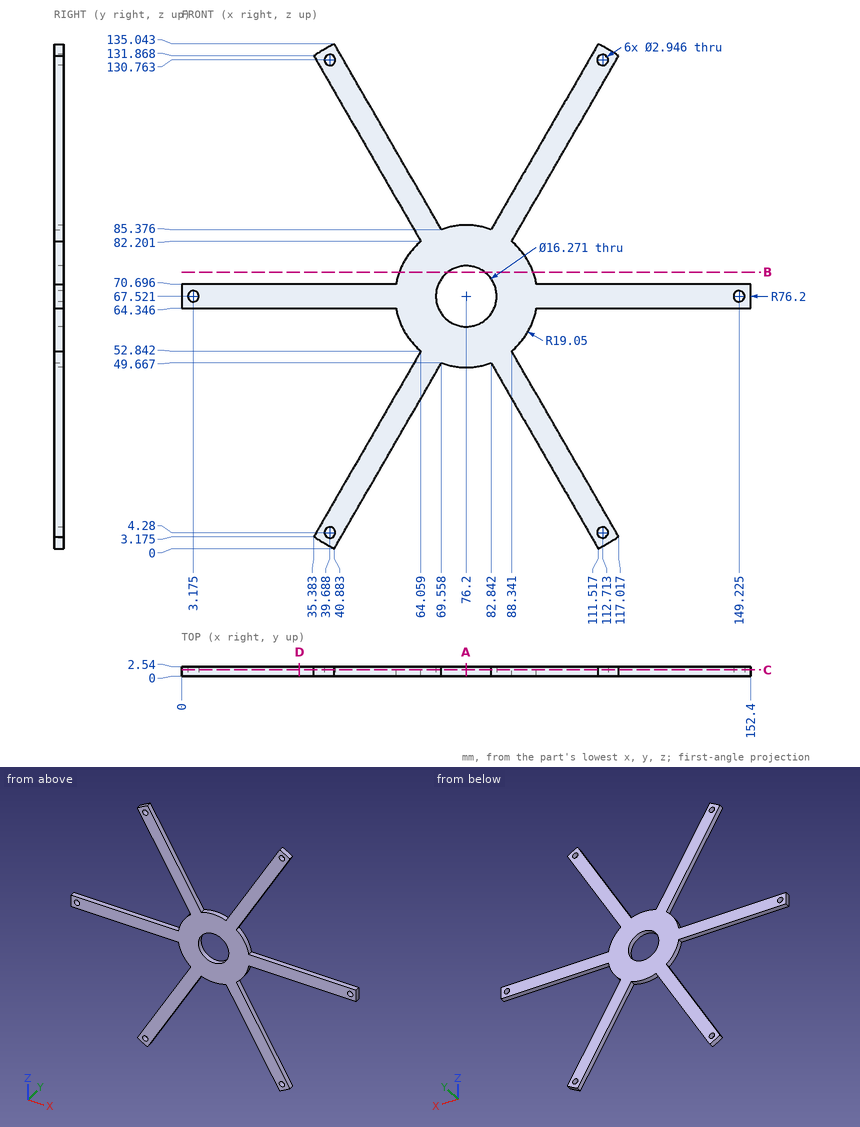
Study the drawing (mm; zero at the part's minimum x, y, z) and answer. Coordinates: 2 decimals unless noted, no trailing zeros. Write each loop counter-clockwise with the first axis right and the second up, starting at its lowest first coordinate (ties: lowest second). Pieces come first, ordered by that corner, then holes. Notation, with made-up numbers: M -1.75,14 L 53.25,14 A21 ccw 53.25,52 Z; hole C 82,37 d5. An arc over 180 degrees is marked long. Use a Markdown table: item, result. Add a question column.
1. Section D-D (x = 31.5) is taken. Give the vertices of the cut face in (y, z), plus the area to 3 significant figures.
2. Section B-B (z = 74) is taken. Give the vertices of the cut face in (x, y) (1 decimal).
3. Section C-C (y = 1.65) is taken. Count the separate pieces of the cut face and the enclosed holes in it, plus the area to 3 significant figures.
4. Section A-A (x = 76.2) is taken. Give the vertices of the cut face in (y, z) (1 decimal).
5. Straight lines are drawn through the part: line 1 along X through (y, z) = (0.65, 68.5) (1 decimal); line 2 along Z through (x, y) = (76.2, 0.6) (1 decimal); line 3 along Z through (x, y) = (25, 0.35). For each, find the intervals that lie inside material, in ascending order. Write a range as [from, to].
6. Given P1, Ø1.3, axis at x = 20.5, y = 1.5, coming from the +Z side; P2, Ø0.8, axis at x = 31.5, y = 1, coming from the -Z side, each flat-ended and moving along its own axis, determine where each tip first touches the part or whether it passes through.
Data:
| question | item | result |
|---|---|---|
| 1 | outline | M 0,64.35 L 2.54,64.35 L 2.54,70.7 L 0,70.7 Z |
| 1 | area | 16.1 mm2 |
| 2 | outline | M 58.3,0 L 71.3,0 L 71.3,2.5 L 58.3,2.5 Z; M 81.1,0 L 94.1,0 L 94.1,2.5 L 81.1,2.5 Z |
| 3 | separate pieces | 1 |
| 3 | enclosed holes | 7 |
| 3 | area | 3,070 mm2 |
| 4 | outline | M 0,48.5 L 2.5,48.5 L 2.5,59.4 L 0,59.4 Z; M 0,75.7 L 2.5,75.7 L 2.5,86.6 L 0,86.6 Z |
| 5 | line 1 | x = [0, 2.1], [4.3, 68.1], [84.3, 148.1], [150.3, 152.4] |
| 5 | line 2 | z = [48.5, 59.4], [75.7, 86.6] |
| 5 | line 3 | z = [64.35, 70.7] |
| 6 | P1 | stops at z = 70.7 |
| 6 | P2 | stops at z = 64.35 |
